```python
from build123d import *

# Parameters (mm, degrees)
F0_W     = 100
F0_H     = 400
F1_DEPTH = 25
F2_W     = 15
F2_H     = 390
F3_DEPTH = 90
F4_R     = 10
F5_DEPTH = 1000
F7_DEPTH = 400
F8_R     = 11.25
F9_DEPTH = 500


with BuildPart() as f1:
    # F0 (on Front) → F1 (new body)
    with BuildSketch(Plane.XZ):
        with Locations((-353.224424, -103.281556)):
            Rectangle(F0_W, F0_H)
    extrude(amount=F1_DEPTH)

    # F2 (on face) → F3 (cut)
    with BuildSketch(Plane.YZ.offset(-303.224424)):
        with Locations((-12.5, -103.281556)):
            Rectangle(F2_W, F2_H)
    extrude(amount=-F3_DEPTH, mode=Mode.SUBTRACT)

    # F4 (on face) → F5 (cut)
    with BuildSketch(Plane(origin=(0, 0, 0), x_dir=(-1, 0, 0), z_dir=(0, 1, 0))):
        with Locations((348.224424, -3.281556)):
            Circle(F4_R)
        with Locations((348.224424, -103.281556)):
            Circle(F4_R)
        with Locations((349.663308, -203.271204)):
            Circle(F4_R)
    extrude(amount=-F5_DEPTH, mode=Mode.SUBTRACT)

    # F6 (on face) → F7 (join)
    with BuildSketch(Plane.XY.offset(96.718444)):
        with BuildLine():
            Line((-403.224424, 0), (-402.187852, 0))
            ThreePointArc((-402.187852, 0), (-436.77333, -12.5), (-402.187852, -25))
            Line((-402.187852, -25), (-403.224424, -25))
            Line((-403.224424, -25), (-403.224424, 0))
        make_face()
        with BuildLine():
            ThreePointArc((-402.187852, -25), (-398.834163, -19.145684), (-397.67006, -12.5))
            ThreePointArc((-397.67006, -12.5), (-398.834163, -5.854316), (-402.187852, 0))
            Line((-402.187852, 0), (-403.224424, 0))
            Line((-403.224424, 0), (-403.224424, -25))
            Line((-403.224424, -25), (-402.187852, -25))
        make_face()
    extrude(amount=-F7_DEPTH)

    # F8 (on face) → F9 (cut)
    with BuildSketch(Plane.XY.offset(96.718444)):
        with Locations((-417.221695, -12.5)):
            Circle(F8_R)
    extrude(amount=-F9_DEPTH, mode=Mode.SUBTRACT)


solid = f1.part
```
Build history of the part. All positions in model axes, mm. A direction names the side the tool comes from. Round coordinates to 2 decimals unless told otherwise and drop trailing zeros. Write each loop counter-clockwise with the first axis right and the second up, starting at its lowest first coordinate (ties: lowest second). Pieces come first, ordered by that corner, then holes.
1) Pin check, flat tips, straight feed: pin 1 (3 mm diameter, centred on x = -415, z = -105, fed in from -Y); pin 2 (8 mm diameter, centred on x = -360, z = -106, fed in from +Y); pin 3 (1.5 mm diameter, centred on y = -6, z = -41.5, fed in from -X). Stop position of each tip, or through.
2) Band-saw the part on A-A, the plane z = -246.5. List the corners of the cut face in (x, y).
3) Band-saw the part on C-C, the plane x = -325.5. List the corners of the cut face in (y, z).
4) Band-saw the part on B-B, the plane y = -12.5. List the corners of the cut face in (x, z), and give its area (3 significant figures).
5) Band-saw the part on D-D, the plane x = -397. List the corners of the cut face in (y, z), and give its area (3 significant figures).
6) 3-axis set-ups, long thin cutter, end or side, ignore diameter. For faces 4 (the flat face through (-348, -13, 91.718)), 5 (the flat face through (-364, -25, -100)), 6 (the flat face through (-364, 0, -100)): which of +Z, -Z, +X, -X, +Y, -Y reach the whole face in a straight line?
7) Drill centre lines: probe 1 along Y at (x, z) = (-348, 13); probe 2 along Z at (x, y) = (-341.5, -10); probe 3 along X at (y, z) = (-12, 44.5). Where is each one in solid material? Low to high.
8) Mould opens along Z. For faces 1 (the cylindrical face through (-428.46, -12.01, -100.48)), 2 (the flat face through (-371, -12, 96.718)), 3 (the flat face through (-393.224, -13, -101)) say: +Z half, -Z half, draft (parallel to the pull), parting line (faces both ways), or undercut.
Ans:
1. pin 1: stops at y = -32.04
1. pin 2: stops at y = 0
1. pin 3: stops at x = -435.91
2. outline: (-402.19, -25) - (-303.22, -25) - (-303.22, -20) - (-393.22, -20) - (-393.22, -5) - (-303.22, -5) - (-303.22, 0) - (-402.19, 0) arc R19.55 ccw (long way) to start; hole circle Ø22.5 at (-417.22, -12.5)
3. outline: (-25, -303.28) - (0, -303.28) - (0, 96.72) - (-25, 96.72) - close; hole (-20, -298.28) - (-5, -298.28) - (-5, 91.72) - (-20, 91.72) - close
4. outline: (-436.77, -303.28) - (-428.47, -303.28) - (-428.47, 96.72) - (-436.77, 96.72) - close; (-405.97, -303.28) - (-303.22, -303.28) - (-303.22, -298.28) - (-393.22, -298.28) - (-393.22, 91.72) - (-303.22, 91.72) - (-303.22, 96.72) - (-405.97, 96.72) - close
4. area: 9,320 mm2
5. outline: (-25, -303.28) - (0, -303.28) - (0, 96.72) - (-25, 96.72) - close
5. area: 10,000 mm2
6. face 4: +X
6. face 5: +Z, -Z, +X, -Y
6. face 6: +Z, -Z, +X, +Y
7. probe 1: y = -25 to -20, -5 to 0
7. probe 2: z = -303.28 to -298.28, 91.72 to 96.72
7. probe 3: x = -436.77 to -428.46, -405.98 to -393.22
8. face 1: draft
8. face 2: +Z half
8. face 3: undercut
